Geometry: see drawing. Coordinates: mm, zero at the bounding-box minimum. A direction names the side the tool comes from. Coordinates: 2 decimals unless noted, no trailing zeros. Loops run counter-clockwise (first coordinate to the right, second up) from the corner with the lowest first, then second, coordinate; pieces in that order, holes last. Notation, with made-up numbers: (32, 28) - (51, 28) arc R21 cw to (51, 51) - close; hole circle Ø5 at (-26.75, -28.75). An arc over 180 degrees is marked (long way). Use one line per item in the form item = value.
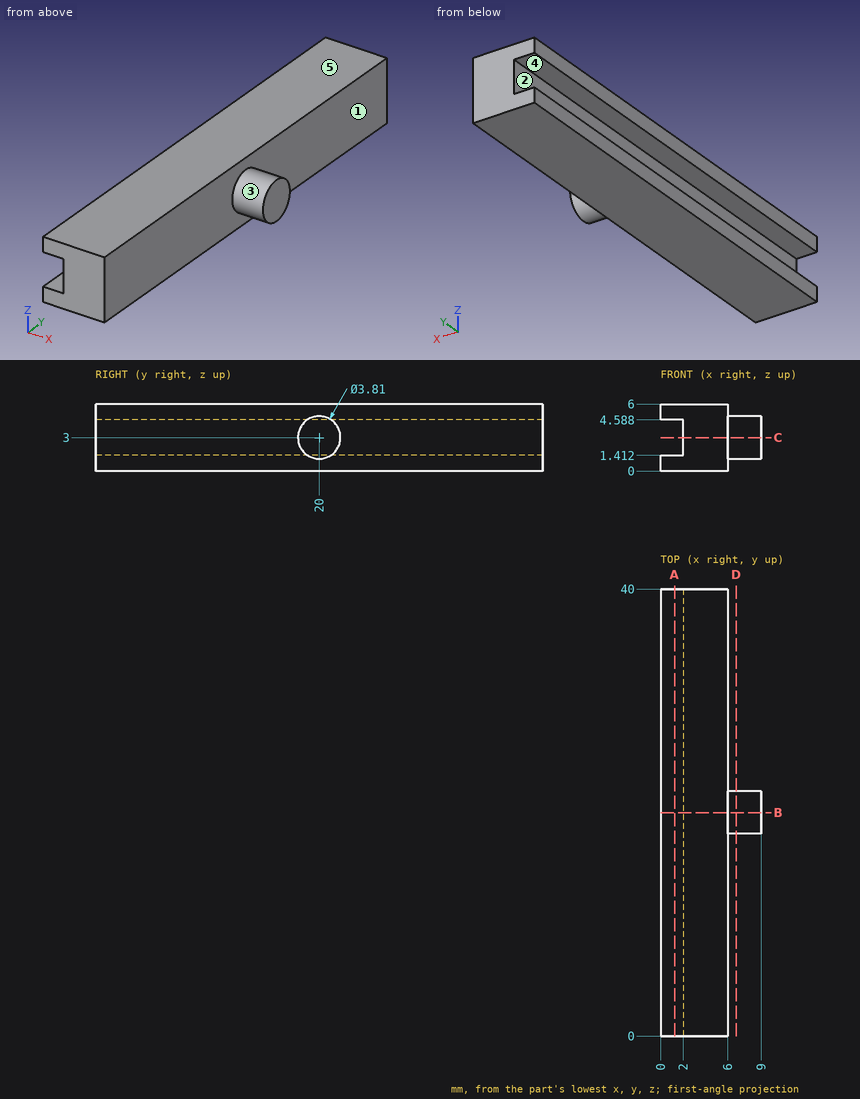
Q1. Pull-direction query (Z, two-part tool) for the marked faces 1, 2 and 3; classes: pulls with the +Z half, pulls with the -Z half, needs draft (parallel to the pull), parting line crosses it, or undercut.
Check values:
face_1 = needs draft
face_2 = undercut
face_3 = parting line crosses it
Q2. First-contact query: P1, Ø1.8, axis at y = 13.5, z = 1.5, coming from the +X side. Flat tip, straight axial feed; report the tip coordinate or a pass-through.
Check values:
P1 = 6
Q3. Cut plane A-A, the plane x = 1.25. Return loops of the section in (y, z), then the cut area to 3 significant figures.
Check values:
outline = (0, 0) - (40, 0) - (40, 1.41) - (0, 1.41) - close; (0, 4.59) - (40, 4.59) - (40, 6) - (0, 6) - close
area = 113 mm²
Q4. Cut plane C-C, the plane z = 3. Return loops of the section in (x, y) (1 decimal).
Check values:
outline = (2, 0) - (6, 0) - (6, 18.1) - (9, 18.1) - (9, 21.9) - (6, 21.9) - (6, 40) - (2, 40) - close
Q5. Cut plane D-D, the plane x = 6.75. Return loops of the section in (y, z) (1 decimal), then the cut area to 3 significant figures.
Check values:
outline = circle Ø3.8 at (20, 3)
area = 11.4 mm²
Q6. Set-up query: the marked faces 4 and 5. Return all of +Z, -Z, +X, -X, +Y, -Y with unobstructed straight access to the full face (end or side cutting, diameter ignored); none if empty.
Check values:
face_4 = -X, +Y, -Y
face_5 = +Z, +X, -X, +Y, -Y
Q7. Cut plane B-B, the plane y = 20. Return loops of the section in (x, z) (1 decimal).
Check values:
outline = (0, 0) - (6, 0) - (6, 1.1) - (9, 1.1) - (9, 4.9) - (6, 4.9) - (6, 6) - (0, 6) - (0, 4.6) - (2, 4.6) - (2, 1.4) - (0, 1.4) - close
Q8. Ray query, line 1 along Z through (x, y) = (1, 7.5); line 2 along X through (y, z) = (30, 1.2); line 3 along X through (y, z) = (26, 4.35). Return the intervals inside material, ascending. Write a range as [from, to].
Check values:
line_1 = [0, 1.41], [4.59, 6]
line_2 = [0, 6]
line_3 = [2, 6]
